Build history of the part. All positions in model axes, mm. A direction names the side the tool comes from. Give positions to 0.01 mm unless a question says otherwise; leave off trailing zeros. Loops run counter-clockwise (first coordinate to the right, second up) from the corner with the lowest first, then second, coordinate; pieces in that order, holes last. Notation, with made-up numbers: (21.25, 50) -> (28.25, 50) arc R34 ccw to (28.25, 88) -> close; hole circle Ø2 at (26, -27). An arc over 180 degrees is marked (long way). One line per question, with ' | ' between items. Start each with the question number.
(1) Slice it at C-C, the plane y = 11. Write the cut outline in (x, z), then the cut area to 3 significant figures.
(2) Flat gauge pins, fed straight in: pin 1 Ø3.5 at (x, z) = (-84, -24.5) entering from +Y; pin 2 Ø2 at (x, z) = (-82, -21) entering from -Y; pin 3 Ø3 at (x, y) = (-90, -2.5) entering from -Z; pin 4 Ø1.5 at (x, z) = (-82, -27) entering from -Y. Where does each tip first touch, or does it go through?
(3) Slice it at A-A, the plane z = -26.5. Write the cut outline in (x, y), then the cut area to 3 significant figures.
(4) Drill centre lines: L1, parallel to Y at x = -83.25, z = -30.5; L2, parallel to Y at x = -84.5, z = -30.5; L3, parallel to Z at x = -88.75, y = -2.5. Where is each one in solid material? Low to high. Write a range as from..to.
(5) Slice it at B-B, the plane x = -84.25. Write the cut outline in (y, z).
(6) Mould opens along Z. For faces 3 (the face through (-92.216, 5, -28)), 4 (the face through (-86, 5, -37.986)), 5 (the face through (-89.516, 11.479, -20.744)), 6 (the face through (-82.318, -2.958, -28.235)) say: pulls with the +Z half, pulls with the -Z half, needs draft (parallel to the pull), parting line crosses it, or undercut.
(7) Slice it at D-D, the plane z = -32.5. Write the cut outline in (x, y), then the cut area to 3 significant figures.
(8) 3-axis set-ups, long thin cutter, end or side, ignore diameter. For faces 1 (the face through (-86, 5, -17.986)), 2 (the face through (-83.186, 11.479, -34.99)): which of +Z, -Z, +X, -X, +Y, -Y reach the whole face in a straight line?
```python
from build123d import *

# Parameters (mm, degrees)
BOSS_EXTRUDE1_DEPTH      = 10
BOSS_EXTRUDE1_DEPTH_BACK = 0.0001
SKETCH2_W                = 11.99345044
SKETCH2_H                = 20
SKETCH3_R                = 4
BOSS_EXTRUDE3_DEPTH      = 6
SKETCH4_R                = 0.5
BOSS_EXTRUDE4_DEPTH      = 3


with BuildPart() as part:
    # Sketch2 → Boss-Extrude1 (new, two sides: drawn at the far end of the back side and taken through both)
    with BuildSketch(Plane(origin=(0, 0, -0.145481973), x_dir=(1, 0, 0), z_dir=(0, 1, 0)).offset(-BOSS_EXTRUDE1_DEPTH_BACK)):
        with Locations((-86.219016819, 27.840556499)):
            Rectangle(SKETCH2_W, SKETCH2_H)
    extrude(amount=BOSS_EXTRUDE1_DEPTH + BOSS_EXTRUDE1_DEPTH_BACK)

    # Sketch3 → Boss-Extrude3 (add)
    with BuildSketch(Plane(origin=(-2.285199676, 0, 0), x_dir=(1, 0, 0), z_dir=(0, 1, 0))):
        with Locations(Location((-83.999243897, 27.714265915, 0), (0, 0, 270))):
            Circle(SKETCH3_R)
    extrude(amount=-BOSS_EXTRUDE3_DEPTH)

    # Sketch4 → Boss-Extrude4 (add)
    with BuildSketch(Plane(origin=(-0.419617144, 10, -0.145481973), x_dir=(1, 0, 0), z_dir=(0, 1, 0))):
        with Locations(Location((-89.592112579, 35.075202762, 0), (0, 0, 270))):
            Circle(SKETCH4_R)
        with Locations(Location((-82.322613513, 35.075202762, 0), (0, 0, 270))):
            Circle(SKETCH4_R)
        with Locations(Location((-82.331654895, 20.533744188, 0), (0, 0, 270))):
            Circle(SKETCH4_R)
        with Locations(Location((-89.592112579, 20.533744188, 0), (0, 0, 270))):
            Circle(SKETCH4_R)
    extrude(amount=BOSS_EXTRUDE4_DEPTH)


solid = part.part
```
Final values:
1) outline: circle Ø1 at (-90.01, -35.22); circle Ø1 at (-90.01, -20.68); circle Ø1 at (-82.75, -20.68); circle Ø1 at (-82.74, -35.22) | area: 3.14 mm2
2) pin 1: y = 10 | pin 2: y = 0 | pin 3: z = -31.04 | pin 4: y = -6
3) outline: (-92.22, 0) -> (-90.1, 0) -> (-90.1, -6) -> (-82.47, -6) -> (-82.47, 0) -> (-80.22, 0) -> (-80.22, 10) -> (-92.22, 10) -> close | area: 166 mm2
4) L1: 0..10 | L2: -6..10 | L3: -30.86..-24.56
5) outline: (-6, -31.16) -> (0, -31.16) -> (0, -37.99) -> (10, -37.99) -> (10, -17.99) -> (0, -17.99) -> (0, -24.27) -> (-6, -24.27) -> close
6) face 3: needs draft | face 4: pulls with the -Z half | face 5: undercut | face 6: parting line crosses it
7) outline: (-92.22, 0) -> (-80.22, 0) -> (-80.22, 10) -> (-92.22, 10) -> close | area: 120 mm2
8) face 1: +Z, +X, -X, +Y, -Y | face 2: +Y
